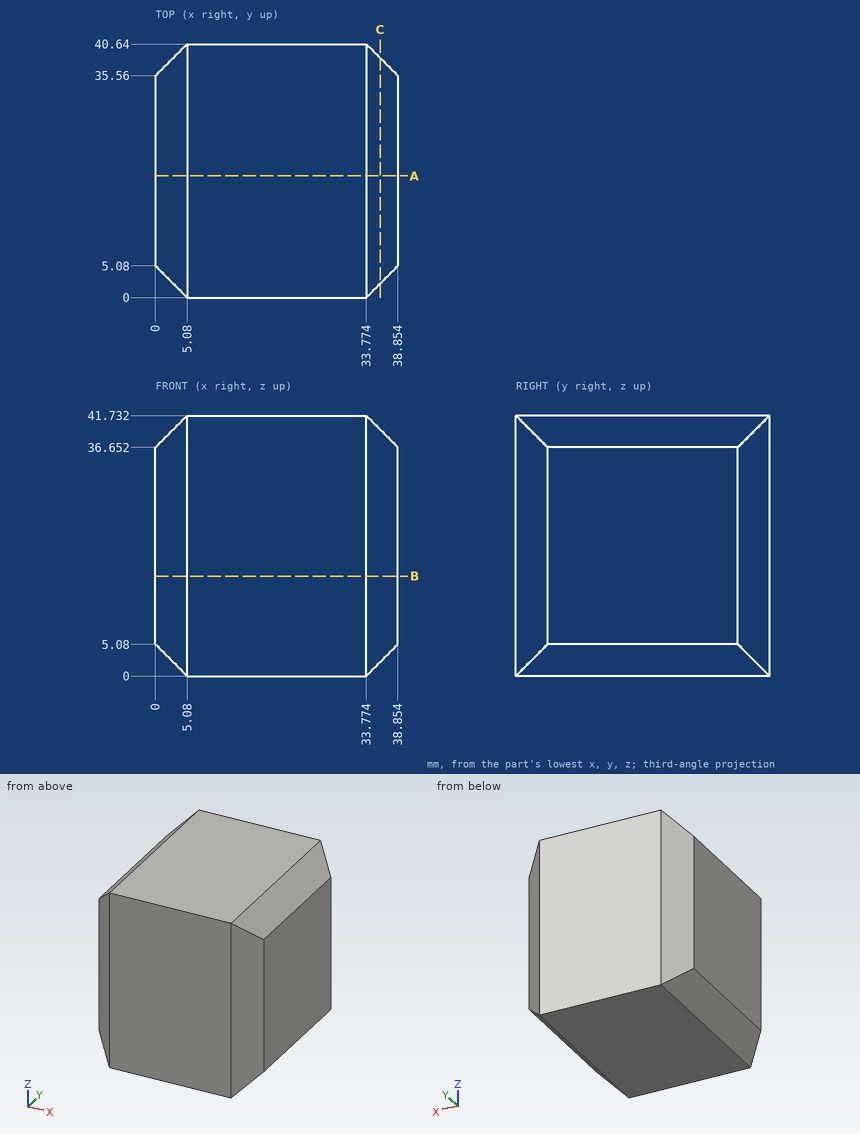
Could you check a few things on this drawing? It's one solid part, dimensions in mm from its lowest x, y, z. Round coordinates to 2 decimals unless told otherwise and drop trailing zeros. Order: outer loops, then holes, each group sorted by start corner. A loop starts at its lowest first (then second) coordinate and runs counter-clockwise, first axis right, second up.
Q1. Imagine slicing it at B-B, the plane z = 16. List the corners of the cut face in (x, y) for me.
Geometry says:
outline: (0, 5.08) - (5.08, 0) - (33.77, 0) - (38.85, 5.08) - (38.85, 35.56) - (33.77, 40.64) - (5.08, 40.64) - (0, 35.56) - close
Q2. Imagine slicing it at C-C, the plane x = 36. List the corners of the cut face in (y, z) for me, then the cut area to 3 significant figures.
Geometry says:
outline: (2.23, 2.23) - (38.41, 2.23) - (38.41, 39.51) - (2.23, 39.51) - close
area: 1,350 mm2
Q3. Imagine slicing it at A-A, the plane y = 19.5. List the corners of the cut face in (x, z) for me.
Geometry says:
outline: (0, 5.08) - (5.08, 0) - (33.77, 0) - (38.85, 5.08) - (38.85, 36.65) - (33.77, 41.73) - (5.08, 41.73) - (0, 36.65) - close
Q4. Please list where these lines run through material, in increasing order: probe 1 along Y at (x, z) = (34, 26.5) (1 decimal); probe 2 along X at (y, z) = (25, 2.5) (1 decimal); probe 3 along X at (y, z) = (36, 19.5) (1 decimal).
Geometry says:
probe 1: y = 0.2 to 40.4
probe 2: x = 2.6 to 36.3
probe 3: x = 0.4 to 38.4
Q5. I'm going to push a flat-ended pin straight in: P1, Ø1, axis at x = 32, z = 13.5, coming from the -Y side. Where does the tip first touch, or does it pass through?
Geometry says:
P1: stops at y = 0
